Design review of the part built by this model. Coordinates are the model's own, in mm. A direction names the side the tool comes from. Coordinates: 2 decimals unless noted, no trailing zeros. Write each loop counter-clockwise with the first axis right and the second up, starting at its lowest first coordinate (ties: lowest second). Pieces come first, ordered by that corner, then holes.
Q1. Insertion check: pin 1 (12 mm diameter, centred on x = -43.5, y = 4, fed in from +Z); pin 2 (6 mm diameter, centred on x = 42.5, y = -8.5, fed in from -Z); pin 3 (6 mm diameter, centred on y = -8.5, z = -1.5, fed in from +X); pin 4 (6 mm diameter, centred on y = -10, z = 38, fed in from +X). Each pin has a flat end and moves straight along its axis. Give the tip position at first contact, or say it passes through.
Q2. Take a section at B-B (z = 12.5). Give the boundary of the cut face in (x, y), and give its area (3 significant figures).
Q3. Take a section at C-C (x = -25). Give the boundary of the cut face in (y, z).
Q4. Mouldability with a two-part tool opening along Y and no side actions: class faces 1 (the flat face through (39, -1, 18.375)), 2 (the flat face through (-4, 44, 6)), 3 (the flat face through (33.024, -1, 7)) as pulls with the +Y half, pulls with the -Y half, needs draft (parallel to the pull), parting line crosses it, or undercut.
Q5. For probe 1 along Y at (x, z) = (24.5, 0); probe 2 along X at (y, z) = (-14, 11); probe 3 along Z at (x, y) = (1, 6), list the stretches that pass through material, from the lowest coordinate up.
Q6. Take a section at A-A (y = 21). Give the boundary of the cut face in (x, z), and give its area (3 significant figures).
Q7. Take a section at D-D (y = -16.5). Give the boundary of the cut face in (x, z), and give its area (3 significant figures).
Q8. Machinability: for faces 4 (the flat face through (36.025, -1, 4)), 5 (the flat face through (39, -1, 21.123)), 6 (the flat face through (-3, 0, -6.625)), which of the approach directions +Z, -Z, +X, -X, +Y, -Y give a long, thin tool a straight path to every point of the face, cutting with its end or side? Answer none if there is none.
```python
from build123d import *

# Parameters (mm, degrees)
F1_DEPTH  = 44
F2_R      = 2.5
F2_R_2    = 2.4725548282
F2_R_3    = 2.4274448112
F3_DEPTH  = 2.748386896
F4_W      = 71.9977971367
F4_H      = 2.4901034832
F4_H_2    = 2.3662897348
F5_DEPTH  = 27.6
F6_R      = 6.9199657135
F7_DEPTH  = 1
F8_R      = 5.6269381347
F9_DEPTH  = 1
F10_R     = 0.5
F11_R     = 2.8344980175
F11_R_2   = 2.7859463521
F12_DEPTH = 65


with BuildPart() as f1:
    # F0 (on Front) → F1 (new body, symmetric)
    with BuildSketch(Plane.XZ):
        Polygon((33.0240737289, -6.6249261405), (-2.9748248395, -6.6249261405), (-2.9748248395, -9.6249261405), (36.0251751605, -9.6249261405), (36.0251751605, 18.3750738595), (48.0240737289, 18.3750738595), (48.0240737289, 21.1234607555), (33.0240737289, 21.1234607555), align=None)
        Polygon((-2.9748248395, -9.6249261405), (-2.9748248395, -6.6249261405), (-38.9737234078, -6.6249261405), (-38.9737234078, 21.1234607555), (-53.9737234078, 21.1234607555), (-53.9737234078, 18.3750738595), (-41.9748248395, 18.3750738595), (-41.9748248395, -9.6249261405), align=None)
    extrude(amount=F1_DEPTH, both=True)

    # F2 (on face) → F3 (cut, through all)
    with BuildSketch(Plane.XY.offset(21.1234607555)):
        with Locations((42.0833444824, -28.976779955)):
            Circle(F2_R)
        with Locations((42.3100408995, 29.0223339752)):
            Circle(F2_R)
        with Locations((-47.6874827498, 29.3740999725)):
            Circle(F2_R)
        with Locations((-47.9141791668, -28.6250139577)):
            Circle(F2_R)
        with Locations((42.192016639, -1.1735668668)):
            Circle(F2_R_2)
        with Locations((-47.8068819294, -1.1735668668)):
            Circle(F2_R_3)
    extrude(amount=-F3_DEPTH, mode=Mode.SUBTRACT)

    # F4 (on face) → F5 (join)
    with BuildSketch(Plane.XY.offset(-6.6249261405)):
        with Locations((-2.9748248395, 42.7549482584)):
            Rectangle(F4_W, F4_H)
        with Locations((-2.9748248395, -42.8168551326)):
            Rectangle(F4_W, F4_H_2)
    extrude(amount=F5_DEPTH)

    # F6 (on face) → F7 (join)
    with BuildSketch(Plane.XY.offset(-6.6249261405)):
        with Locations((-3.1422167085, 0.3347826132)):
            Circle(F6_R)
    extrude(amount=F7_DEPTH)

    # F8 (on face) → F9 (cut)
    with BuildSketch(Plane.XY.offset(-5.6249261405)):
        with Locations((-3.1422167085, 0.3347826132)):
            Circle(F8_R)
    extrude(amount=-F9_DEPTH, mode=Mode.SUBTRACT)

    # F10
    f10_edges = [f1.edges().sort_by_distance(p)[0] for p in [
        (-10.062182, 0.334783, -5.624926),
        (-8.769155, 0.334783, -5.624926),
    ]]
    fillet(f10_edges, radius=F10_R)

    # F11 (on face) → F12 (join)
    with BuildSketch(Plane.XY.offset(-6.6249261405)):
        with Locations((-20.3835200518, 15.5673911795)):
            Circle(F11_R)
        with Locations((-20.3835200518, -17.7434775978)):
            Circle(F11_R_2)
    extrude(amount=F12_DEPTH)


solid = f1.part
```
Response:
1. pin 1: stops at z = 21.12
1. pin 2: stops at z = 18.38
1. pin 3: stops at x = 36.03
1. pin 4: passes through
2. outline: (-41.97, -44) - (36.03, -44) - (36.03, 44) - (-41.97, 44) - close; circle Ø5.67 at (-20.38, 15.57); circle Ø5.57 at (-20.38, -17.74); hole (-38.97, -41.63) - (33.02, -41.63) - (33.02, 41.51) - (-38.97, 41.51) - close
2. area: 927 mm2
3. outline: (-44, -9.62) - (44, -9.62) - (44, 20.98) - (41.51, 20.98) - (41.51, -6.62) - (-41.63, -6.62) - (-41.63, 20.98) - (-44, 20.98) - close
4. face 1: needs draft
4. face 2: pulls with the +Y half
4. face 3: undercut
5. probe 1: y = -44 to -41.63, 41.51 to 44
5. probe 2: x = -41.97 to -38.97, 33.02 to 36.03
5. probe 3: z = -9.62 to -6.62
6. outline: (-53.97, 18.38) - (-41.97, 18.38) - (-41.97, -9.62) - (36.03, -9.62) - (36.03, 18.38) - (48.02, 18.38) - (48.02, 21.12) - (33.02, 21.12) - (33.02, -6.62) - (-38.97, -6.62) - (-38.97, 21.12) - (-53.97, 21.12) - close
6. area: 467 mm2
7. outline: (-53.97, 18.38) - (-41.97, 18.38) - (-41.97, -9.62) - (36.03, -9.62) - (36.03, 18.38) - (48.02, 18.38) - (48.02, 21.12) - (33.02, 21.12) - (33.02, -6.62) - (-17.89, -6.62) - (-17.89, 58.38) - (-22.88, 58.38) - (-22.88, -6.62) - (-38.97, -6.62) - (-38.97, 21.12) - (-53.97, 21.12) - close
7. area: 791 mm2
8. face 4: -Z, +X, +Y, -Y
8. face 5: +Z, +X, +Y, -Y
8. face 6: +Z
